Geometry: see drawing. Coordinates: mm, zero at the bounding-box minimum. Give positions to 0.01 mm unless a question says otherwise; leave off trailing zeros. Loops run counter-clockwise (first coordinate to the right, second up) from the corner with the lowest first, then second, coordinate; pieces in that order, holes last. Notation, with made-up numbers: (-1, -24.5) -> (17, -24.5) arc R29 ccw to (17, 1.5) -> close; hole circle Ø11 at (-2.75, 84.25). An arc over 180 degrees is marked (long way). Return JSON: item names as keys, results as strings. Group by question number.
(1) Draft query along Y for the marked faces 1, 2 and 3. Return one class per face: released by +Y, released by -Y, zero draft, split by the parting line, or undercut.
(2) Cut plane C-C on z = 10. Return loops of the section in (x, y).
(3) Cut plane A-A on y = 23. Return loops of the section in (x, z), then the cut area to 3 significant figures.
(4) Cut plane B-B on x = 29. Return loops of the section in (y, z) (1 decimal), then the cut area to 3 significant figures.
(5) Ray query, line 1 (X direction, y = 23.5, z = 17); line 2 (Y direction, x = 36, z = 23.5) (1 decimal); line 3 (X direction, y = 18, z = 18) (1 decimal). Return the intervals inside material, ascending. Write a range as from..to.
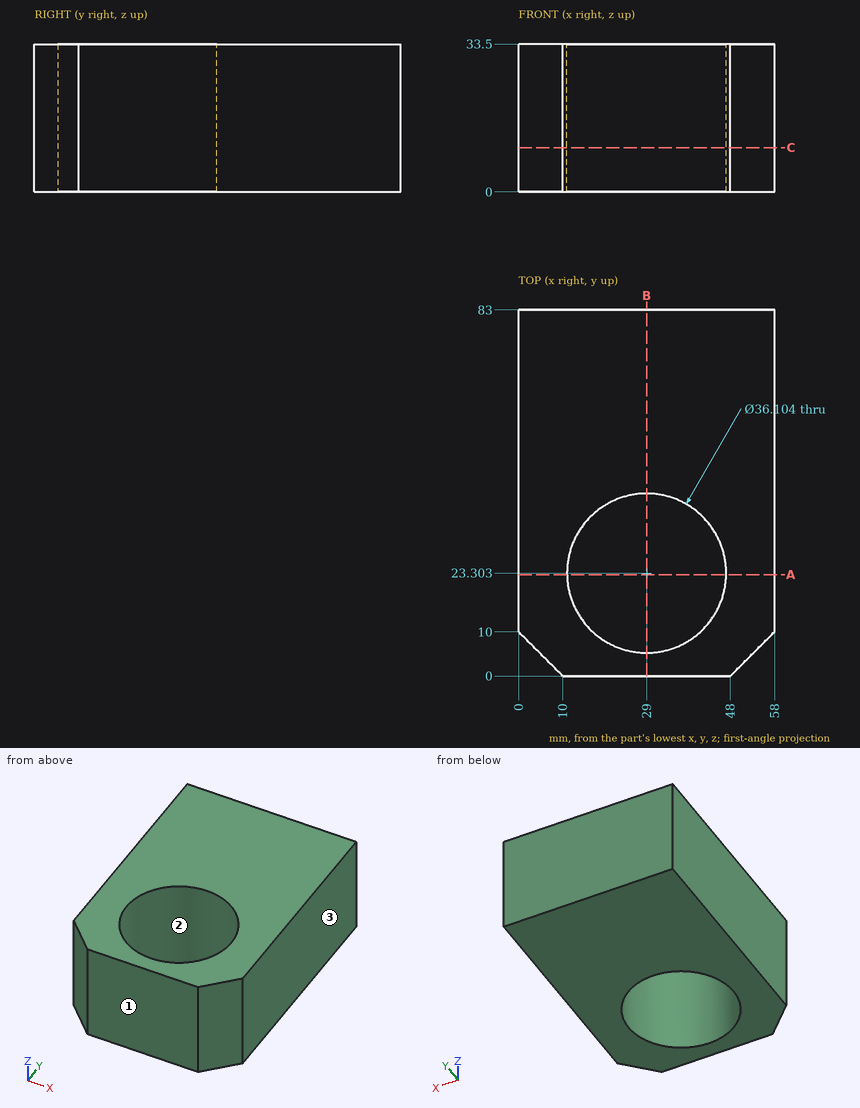
Answers:
{
 "1": {"face 1": "released by -Y", "face 2": "undercut", "face 3": "zero draft"},
 "2": {"outline": "(0, 10) -> (10, 0) -> (48, 0) -> (58, 10) -> (58, 83) -> (0, 83) -> close; hole circle Ø36.1 at (29, 23.3)"},
 "3": {"outline": "(0, 0) -> (10.95, 0) -> (10.95, 33.5) -> (0, 33.5) -> close; (47.05, 0) -> (58, 0) -> (58, 33.5) -> (47.05, 33.5) -> close", "area": "734 mm²"},
 "4": {"outline": "(0, 0) -> (5.3, 0) -> (5.3, 33.5) -> (0, 33.5) -> close; (41.4, 0) -> (83, 0) -> (83, 33.5) -> (41.4, 33.5) -> close", "area": "1,570 mm²"},
 "5": {"line 1": "0..10.95, 47.05..58", "line 2": "0..6.7, 39.9..83", "line 3": "0..11.7, 46.3..58"}
}
